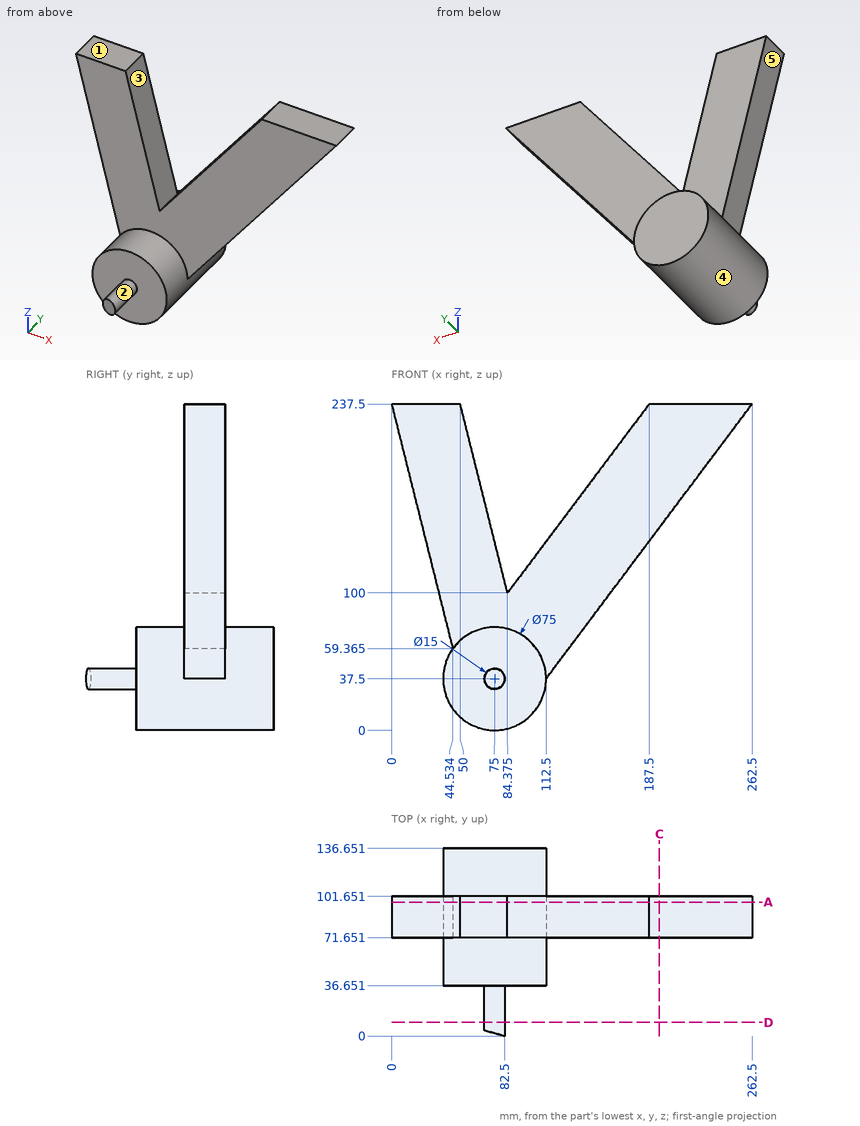
Study the drawing (mm; zero at the part's minimum x, y, z) and answer. A direction names the side the tool comes from. Give positions to 0.01 mm unless a question says otherwise; leave off trailing zeros. Write each loop counter-clockwise with the first axis right and the second up, starting at its lowest first coordinate (ties: lowest second). Pieces come first, ordered by that corner, then holes. Notation, with made-up numbers: (71, 57) - (123, 57) arc R15 ccw to (123, 82) - close; hole circle Ø6 at (-6, -2). An arc over 180 degrees is marked (long way). One line per question, with ' | ' between items. Start each with the question number.
1. Section D-D, the plane y = 10 is taken. Determine the outline of the cut face in (x, z).
2. Given P1, Ø10, axis at x = 177.5, y = 93, coming from the -Z side; P2, Ø12, axis at x = 191.5, y = 104.5, coming from the -Z side (1 decimal); P3, Ø8, axis at y = 43, z = 44, coming from the -X side, each flat-ended and moving along its own axis, determine where each tip first touches the part or whether it passes through.
3. Section A-A, the plane y = 97.5 is taken. Determine the outline of the cut face in (x, z) (1 decimal), then the cut area to 3 significant figures.
4. Determine the mould class of the marked faces 3, 4 and 5 for opening direction X: +X half, -X half, draft (parallel to the pull), parting line (faces both ways), or undercut.
5. Section C-C, the plane x = 195 is taken. Determine the outline of the cut face in (y, z), then the cut area to 3 significant figures.
6. Straight lines are drawn through the part: line 1 (Y direction, x = 54, z = 13.5); line 2 (X direction, y = 77, z = 118) (1 decimal); line 3 (X direction, y = 93.5, z = 208) (1 decimal). For each, find the intervals that lie inside material, in ascending order.
7. For the marked faces 1 and 2, determine the directions among +Z, -Z, +X, -X, +Y, -Y from which every point of the face is accessible in a straight line to the end or side of a thin tool.
Result:
1) outline: circle Ø15 at (75, 37.5)
2) P1: stops at z = 117.5 | P2: stops at z = 135.8 | P3: stops at x = 37.58
3) outline: (0, 237.5) - (44.5, 59.4) arc R37.5 ccw (long way) to (112.5, 37.5) - (262.5, 237.5) - (187.5, 237.5) - (84.4, 100) - (50, 237.5) - close | area: 25,400 mm2
4) face 3: undercut | face 4: parting line | face 5: -X half
5) outline: (71.65, 147.5) - (101.65, 147.5) - (101.65, 237.5) - (71.65, 237.5) - close | area: 2,700 mm2
6) line 1: y = 36.65 to 136.65 | line 2: x = 29.9 to 79.9, 97.9 to 172.9 | line 3: x = 7.4 to 57.4, 165.4 to 240.4
7) face 1: +Z, +X, -X, +Y, -Y | face 2: -Y
